from build123d import *

# Parameters (mm, degrees)
SKETCH1_W           = 20
SKETCH1_H           = 40
BOSS_EXTRUDE1_DEPTH = 3
BOSS_EXTRUDE2_DEPTH = 10
SKETCH4_W           = 20
SKETCH4_H           = 40
BOSS_EXTRUDE3_DEPTH = 3


with BuildPart() as part:
    # Sketch1 → Boss-Extrude1 (new body)
    with BuildSketch(Plane(origin=(0, 0, 0), x_dir=(1, 0, 0), z_dir=(0, 1, 0))):
        Rectangle(SKETCH1_W, SKETCH1_H)
    extrude(amount=BOSS_EXTRUDE1_DEPTH)

    # Sketch2 → Boss-Extrude2 (add)
    with BuildSketch(Plane(origin=(0, 3, 0), x_dir=(1, 0, 0), z_dir=(0, 1, 0))):
        Polygon((-10, -20), (10, -20), (10, -4), (7, -4), (7, 0), (7, 4), (10, 4), (10, 20), (-10, 20), align=None)
    extrude(amount=BOSS_EXTRUDE2_DEPTH)

    # Sketch4 → Boss-Extrude3 (add)
    with BuildSketch(Plane(origin=(0, 13, 0), x_dir=(1, 0, 0), z_dir=(0, 1, 0))):
        Rectangle(SKETCH4_W, SKETCH4_H)
    extrude(amount=BOSS_EXTRUDE3_DEPTH)


solid = part.part
CAD build for the part. Positions are in the model's coordinates, mm. A direction names the side the tool comes from. Give positions to 0.01 mm unless a question says otherwise; leave off trailing zeros. Write each loop counter-clockwise with the first axis right and the second up, starting at its lowest first coordinate (ties: lowest second). Pieces come first, ordered by that corner, then holes. Notation, with made-up numbers: (58.5, 64.25) -> (82.5, 64.25) arc R9 ccw to (82.5, 79.25) -> close; hole circle Ø1 at (24.25, -30.75). An arc over 180 degrees is marked (long way). Return JSON: item names as keys, results as strings.
Item 1: Drop a flat-ended pin along its axis: pin 1 (9 mm diameter, centred on y = 10.5, z = 1, fed in from +X). Give the stop position or say it passes through.
Answer below:
{"pin 1": "stops at x = 10"}
Item 2: Band-saw the part on A-A (x = 8). List the corners of the cut face in (y, z).
Answer below:
{"outline": "(0, -20) -> (16, -20) -> (16, 20) -> (0, 20) -> close; hole (3, -4) -> (13, -4) -> (13, 4) -> (3, 4) -> close"}
Item 3: Drill centre line: probe 1 along X at (y, z) = (5.25, 1). Where is it in solid material? Low to high.
Answer below:
{"probe 1": "x = -10 to 7"}
Item 4: Tool access for faces 1 (the flat face through (-10, 8, 0)), 2 (the flat face through (7, 8, 0)): list every direction of +Z, -Z, +X, -X, +Y, -Y with a clear straight run to the whole face (end or side of a thin tool).
Answer below:
{"face 1": "+Z, -Z, -X, +Y, -Y", "face 2": "+X"}
Item 5: Two-plate mould, pull along Y, no slides. Class faces 3 (the flat face through (0, 8, 20)), 4 (the flat face through (9, 8, 4)), 5 (the flat face through (0, 16, 0)): +Y half, -Y half, draft (parallel to the pull), parting line (faces both ways), or undercut.
Answer below:
{"face 3": "draft", "face 4": "undercut", "face 5": "+Y half"}
Item 6: Band-saw the part on C-C (z = -3). List the corners of the cut face in (x, y).
Answer below:
{"outline": "(-10, 0) -> (10, 0) -> (10, 3) -> (7, 3) -> (7, 13) -> (10, 13) -> (10, 16) -> (-10, 16) -> close"}
Item 7: Band-saw the part on B-B (y = 12.25). List the corners of the cut face in (x, z), then the cut area to 3 significant figures.
Answer below:
{"outline": "(-10, -20) -> (10, -20) -> (10, -4) -> (7, -4) -> (7, 4) -> (10, 4) -> (10, 20) -> (-10, 20) -> close", "area": "776 mm2"}
